```python
from build123d import *

# Parameters (mm, degrees)
BOSS_EXTRUDE1_DEPTH = 7.874
SKETCH4_R           = 1.778
CUT_EXTRUDE2_DEPTH  = 20.828
CUT_EXTRUDE3_START  = -6.35
SKETCH5_R           = 1.778
CUT_EXTRUDE3_DEPTH  = 6.35


with BuildPart() as part:
    # Sketch1 → Boss-Extrude1 (new body)
    with BuildSketch(Plane(origin=(0, 0, 0), x_dir=(0, 0, -1), z_dir=(1, 0, 0))):
        Polygon((-10.547521943, 32.599346848), (-10.547521943, 7.199346848), (-36.963521943, 7.199346848), (-36.963521943, 8.723346848), (-15.627521943, 8.723346848), (-15.627521943, 27.558210738), (-41.027521943, 27.558210738), (-41.027521943, 32.599346848), align=None)
    extrude(amount=-BOSS_EXTRUDE1_DEPTH)

    # Sketch4 → Cut-Extrude2 (cut)
    with BuildSketch(Plane(origin=(0, 0, 0), x_dir=(1, 0, 0), z_dir=(0, 1, 0))):
        with Locations(Location((-5.23875, -18.631071943, 0), (0, 0, 90))):
            Circle(SKETCH4_R)
        with Locations(Location((-5.23875, -34.125071943, 0), (0, 0, 90))):
            Circle(SKETCH4_R)
    extrude(amount=CUT_EXTRUDE2_DEPTH, mode=Mode.SUBTRACT)

    # Sketch5 → Cut-Extrude3 (cut)
    with BuildSketch(Plane(origin=(0, 32.599346848, 0), x_dir=(1, 0, 0), z_dir=(0, 1, 0)).offset(CUT_EXTRUDE3_START)):
        with Locations(Location((-5.23875, -18.631071943, 0), (0, 0, 90))):
            Circle(SKETCH5_R)
        with Locations(Location((-5.23875, -37.681071943, 0), (0, 0, 270))):
            Circle(SKETCH5_R)
    extrude(amount=CUT_EXTRUDE3_DEPTH, mode=Mode.SUBTRACT)


solid = part.part
```
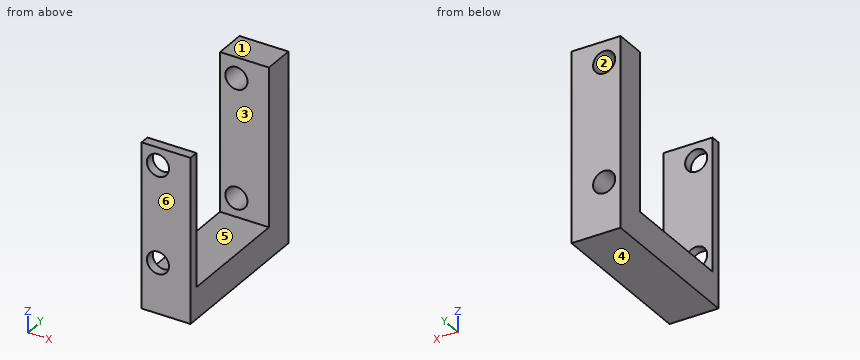
Geometry: final body of the model. Coordinates: model frame, mm. Face numbers are marked on the shaded views. A direction names the side the tool comes from. Round coordinates to 2 decimals unless told otherwise and drop trailing zeros. Loops run counter-clockwise (first coordinate to the right, second up) from the corner with the lowest first, then second, coordinate; pieces in that order, holes last. Notation, with made-up numbers: (48.25, 77.5) -> (54.25, 77.5) arc R11 cw to (54.25, 94.5) -> close; hole circle Ø9 at (59.25, -15). An arc over 180 degrees is marked (long way). Use one line per item in the form item = value.
Item 1: Cut plane A-A on z = 16. Output: boundary loops of the cut face in (x, y).
Evaluation:
outline = (-7.87, 7.2) -> (0, 7.2) -> (0, 8.72) -> (-7.87, 8.72) -> close; (-7.87, 27.56) -> (0, 27.56) -> (0, 32.6) -> (-7.87, 32.6) -> close
Item 2: Cut plane D-D on z = 33. Output: boundary loops of the cut face in (x, y), then the cut area to 3 significant figures.
Evaluation:
outline = (-7.87, 7.2) -> (-6.62, 7.2) -> (-6.62, 8.72) -> (-7.87, 8.72) -> close; (-7.87, 27.56) -> (0, 27.56) -> (0, 32.6) -> (-7.87, 32.6) -> close; (-3.86, 7.2) -> (0, 7.2) -> (0, 8.72) -> (-3.86, 8.72) -> close
area = 47.5 mm2
Item 3: Contact query for flat-ended pins moving along their axis: pin 1 Ø4 at (x, y) = (-7, 12.5) entering from +Z; pin 2 Ø0.8 at (x, y) = (-4, 7.5) entering from +Z; pin 3 Ø3 at (x, z) = (-5.24, 34.13) entering from -Y. Output: stop coordinate, or through.
Evaluation:
pin_1 = 15.63
pin_2 = 36.96
pin_3 = 27.56
Item 4: Access query for the marked faces 1, 2 and 3. Directions: +Z, -Z, +X, -X, +Y, -Y. A direction counts if a zero-diameter tool reaches every point of the face in a straight line with its end or side. Return the directions, or none.
Evaluation:
face_1 = +Z, +X, -X, +Y, -Y
face_2 = +Y
face_3 = +Z, +X, -X
Item 5: Material intervals for probe 1 along Y at (x, z) = (-2.25, 36.5); probe 2 along Z at (x, y) = (-1, 19.25); probe 3 along X at (y, z) = (30.5, 37.5), sorted ascending.
Evaluation:
probe_1 = 7.2 to 8.72, 27.56 to 32.6
probe_2 = 10.55 to 15.63
probe_3 = -7.87 to -7.01, -3.47 to 0
Item 6: Cut plane B-B on x = -1.75. Output: boundary loops of the cut face in (y, z).
Evaluation:
outline = (7.2, 10.55) -> (32.6, 10.55) -> (32.6, 41.03) -> (27.56, 41.03) -> (27.56, 15.63) -> (8.72, 15.63) -> (8.72, 36.96) -> (7.2, 36.96) -> close
Item 7: Cut plane C-C on x = -4. Output: boundary loops of the cut face in (y, z), then the cut area to 3 significant figures.
Evaluation:
outline = (7.2, 10.55) -> (32.6, 10.55) -> (32.6, 17.36) -> (27.56, 17.36) -> (27.56, 15.63) -> (8.72, 15.63) -> (8.72, 17.36) -> (7.2, 17.36) -> close; (7.2, 19.91) -> (8.72, 19.91) -> (8.72, 32.85) -> (7.2, 32.85) -> close; (7.2, 35.4) -> (8.72, 35.4) -> (8.72, 36.96) -> (7.2, 36.96) -> close; (27.56, 19.91) -> (32.6, 19.91) -> (32.6, 36.41) -> (27.56, 36.41) -> close; (27.56, 38.96) -> (32.6, 38.96) -> (32.6, 41.03) -> (27.56, 41.03) -> close
area = 256 mm2
Item 8: Draft query along Y for the marked faces 4, 5 and 6. Return one class per face: released by +Y, released by -Y, zero draft, split by the parting line, or undercut.
Evaluation:
face_4 = zero draft
face_5 = undercut
face_6 = released by -Y
